Job drawing, mm, ordinate dimensions from the low corner. One solid piece. Coordinates: 2 decimals unless noted, no trailing zeros. Write each loop counter-clockwise with the first axis right and the second up, starting at its lowest first coordinate (ties: lowest second). Pieces come first, ordered by that corner, then holes. Notation, with made-up numbers: (16, 76.25) - (71, 76.25) arc R17 cw to (71, 101.25) - close; hole circle Ø2 at (18, -15). An arc over 180 degrees is marked (long way). Put each result on its own line as item: value. Start each with the question number.
1. Drop flat-ended pins along their axis: P1, Ø1.5, axis at y = 40, z = 9.5, coming from the -X side; P2, Ø5, axis at x = 47, z = 8.5, coming from the +Y side; P3, Ø1.5, axis at y = 74, z = 6, coming from the -X side (1 decimal). Give the stop position or say it passes through.
2. Drill centre lines: L1, parallel to X at y = 86, z = 0.5; L2, parallel to X at y = 89, z = 3.25; L3, parallel to Y at x = 24, z = 9.25 (1 decimal). Where is each one in solid material? Low to high. Write a range as from..to.
3. Saw through at C-C, the plane y = 27. Write the cut outline in (x, z), plus the area to 3 significant figures.
4. Saw through at B-B, the plane x = 64.5. Write the cut outline in (y, z).
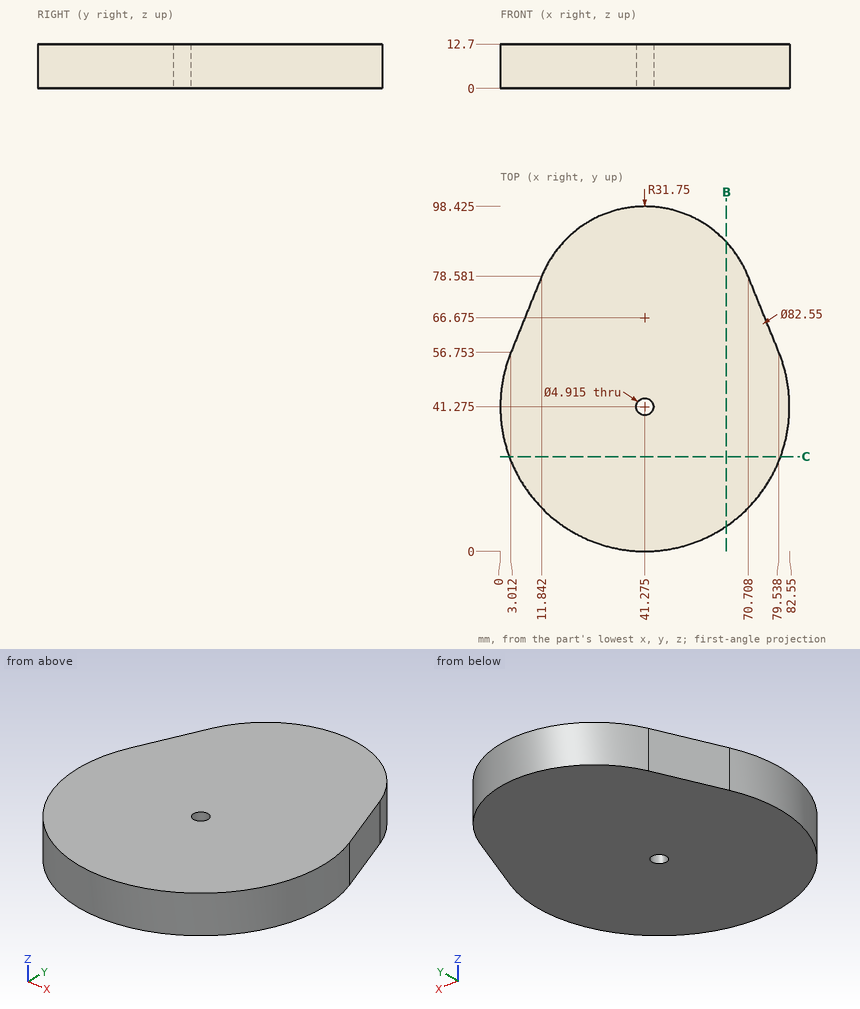
Final values:
1. P1: stops at x = 0
1. P2: stops at y = 98.26
1. P3: stops at x = 9.7
2. L1: x = 16.08..66.47
2. L2: x = 18.7..63.85
2. L3: y = 3.8..93.3
3. outline: (2.55, 0) - (80, 0) - (80, 12.7) - (2.55, 12.7) - close
3. area: 984 mm²
4. outline: (7.15, 0) - (88.32, 0) - (88.32, 12.7) - (7.15, 12.7) - close
